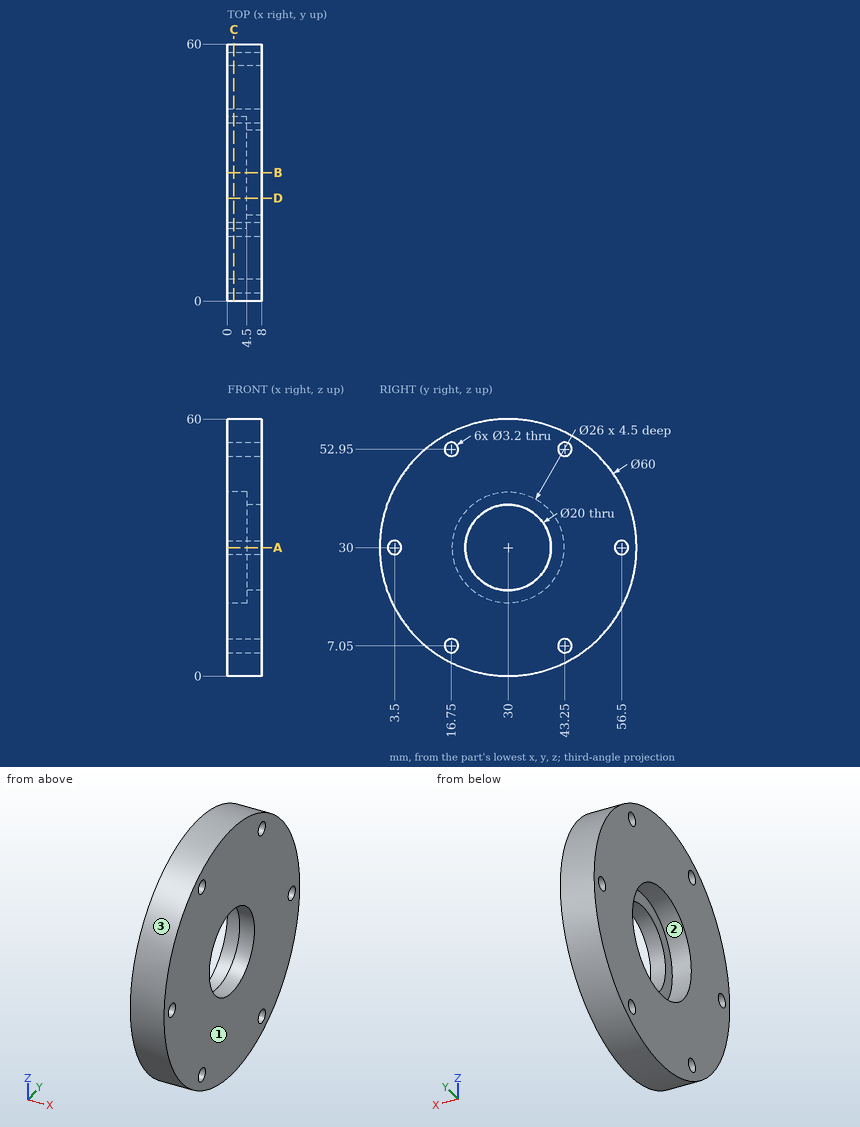
Can you work these out from the drawing? Everything is in mm from the part's minimum corner. Coordinates: 2 decimals unless noted, no trailing zeros. Loops run counter-clockwise (first coordinate to the right, second up) from the corner with the lowest first, then second, coordinate; pieces in that order, holes last.
1. For P1, Ø3, axis at y = 43.25, z = 7.05, coming from the +X side; P2, Ø1, axis at x = 1, z = 9, coming from the +Y side; P3, Ø5, axis at y = 43.25, z = 52.95, coming from the -X side; P4, Ø2, axis at x = 6, y = 51, coming from the -Z side, each with a flat end and sliding along its axis, tell me the tip position at first contact or that it passes through.
2. Imagine slicing it at D-D, the plane y = 24. Please give me the cut outline in (x, z).
3. I need wall thicknesses on L1, parallel to Y at x = 1.25, z = 53; L2, parallel to Z at x = 6.6, y = 30; L3, parallel to Z at x = 2.75, y = 29. Which ranges of each line are inside material? Lowest first, please.
4. Imagine slicing it at B-B, the plane y = 30. Please give me the cut outline in (x, z).
5. Imagine slicing it at A-A, the plane z = 30. Please give me the cut outline in (x, y), and give its area (3 significant figures).
6. If we mould it in two halves opening along Y, with no side actions, what happens to the marked faces 1, 2 and 3? For each: pulls with the +Y half, pulls with the -Y half, needs draft (parallel to the pull), parting line crosses it, or undercut.
7. Imagine slicing it at C-C, the plane x = 1.5. Please give me the cut outline in (y, z), and give its area (3 significant figures).
Taken from the geometry:
1. P1: passes through
1. P2: stops at y = 51.9
1. P3: stops at x = 0
1. P4: stops at z = 7.64
2. outline: (0, 0.61) - (8, 0.61) - (8, 22) - (4.5, 22) - (4.5, 18.47) - (0, 18.47) - close; (0, 41.53) - (4.5, 41.53) - (4.5, 38) - (8, 38) - (8, 59.39) - (0, 59.39) - close
3. L1: y = 10.74 to 15.15, 18.35 to 41.65, 44.85 to 49.26
3. L2: z = 0 to 20, 40 to 60
3. L3: z = 0.02 to 17.04, 42.96 to 59.98
4. outline: (0, 0) - (8, 0) - (8, 20) - (4.5, 20) - (4.5, 17) - (0, 17) - close; (0, 43) - (4.5, 43) - (4.5, 40) - (8, 40) - (8, 60) - (0, 60) - close
5. outline: (0, 0) - (8, 0) - (8, 1.9) - (0, 1.9) - close; (0, 5.1) - (8, 5.1) - (8, 20) - (4.5, 20) - (4.5, 17) - (0, 17) - close; (0, 43) - (4.5, 43) - (4.5, 40) - (8, 40) - (8, 54.9) - (0, 54.9) - close; (0, 58.1) - (8, 58.1) - (8, 60) - (0, 60) - close
5. area: 242 mm2
6. face 1: needs draft
6. face 2: undercut
6. face 3: parting line crosses it
7. outline: circle Ø60 at (30, 30); hole circle Ø3.2 at (3.5, 30); hole circle Ø3.2 at (16.75, 7.05); hole circle Ø3.2 at (16.75, 52.95); hole circle Ø26 at (30, 30); hole circle Ø3.2 at (43.25, 7.05); hole circle Ø3.2 at (43.25, 52.95); hole circle Ø3.2 at (56.5, 30)
7. area: 2,250 mm2
